Model file for the job. Use its own axes, mm. A direction names the side the tool comes from. Round coordinates to 2 decimals unless told otherwise and drop trailing zeros. Order: outer loops, then holes, each group sorted by start corner. A loop starts at its lowest first (then second) coordinate and runs counter-clockwise, first axis right, second up. Notation, with made-up numbers: (57.25, 86.5) - (70.25, 86.5) arc R20 ccw to (70.25, 120.5) - close; hole circle Ø1 at (75, -13). An arc over 180 degrees is marked (long way). Write item = value, one per line. Start each with the question number.
from build123d import *

# Parameters (mm, degrees)
F0_R     = 12.5
F1_DEPTH = 8.5
F2_R     = 10
F3_DEPTH = 5
F4_R     = 8
F5_DEPTH = 13.501
F6_SIZE  = 0.2


with BuildPart() as f1:
    # F0 (on Top) → F1 (new body)
    with BuildSketch(Plane.XY):
        Circle(F0_R)
    extrude(amount=F1_DEPTH)

    # F2 (on face) → F3 (join)
    with BuildSketch(Plane.XY.offset(8.5)):
        Circle(F2_R)
    extrude(amount=F3_DEPTH)

    # F4 (on face) → F5 (cut, through all)
    with BuildSketch(Plane.XY.offset(13.5)):
        Circle(F4_R)
    extrude(amount=-F5_DEPTH, mode=Mode.SUBTRACT)

    # F6
    f6_edges = [f1.edges().sort_by_distance(p)[0] for p in [
        (-10, 0, 13.5),
        (-8, 0, 13.5),
        (-12.5, 0, 8.5),
        (-10, 0, 8.5),
        (-12.5, 0, 0),
        (-8, 0, 0),
    ]]
    chamfer(f6_edges, length=F6_SIZE)


solid = f1.part
Item 1: Which spindle directions (+Z, -Z, +X, -X, +Y, -Y) get a long thin tool onto all of the face, cutting with end or side? Do faces 1 (the face through (-7.35, 7.35, 8.5)), 2 (the face through (-6, -6, 13.5)). Say none if no direction does.
Item 2: Mould opens along X. For faces 3 (the face through (8, -3, 0)), 4 (the face through (-1.73, -7.81, 6.84)), 5 (the face through (-2.17, -9.76, 10.97)) say: +X half, -X half, draft (parallel to the pull), parting line (faces both ways), or undercut.
Item 3: Drop flat-ended pins along their axis: pin 1 (6 mm diameter, centred on x = 10, z = 9.5, fed in from -Y); pin 2 (2 mm diameter, centred on x = 10, z = 9, fed in from +Y); pin 3 (5 mm diameter, centred on x = -9, z = 7, fed in from -Y). Give the stop position or say it passes through.
Item 4: Saw through at D-D, the plane z = 5.25. Give the cut face in (x, y).
Item 5: Probe L1, parallel to Y at x = 0, z = 4.75; L2, parallel to Y at x = 0, z = 8.75; L3, parallel to X at y = 4.25, z = 2.5. List the from-to ranges inside material, lowest first.
Item 6: Saw through at A-A, the plane y = 0. Give the cut face in (x, z), then the cut area to 3 significant figures.
Item 7: Saw through at C-C, the plane z = 11.5. Give the cut face in (x, y).
Check sheet entries:
q1.face_1 = +Z
q1.face_2 = +Z, +X, -X, +Y, -Y
q2.face_3 = draft
q2.face_4 = undercut
q2.face_5 = parting line
q3.pin_1 = -10.18
q3.pin_2 = 8.37
q3.pin_3 = -10.68
q4.outline = circle Ø25 at (0, 0); hole circle Ø16 at (0, 0)
q5.L1 = -12.5 to -8, 8 to 12.5
q5.L2 = -10 to -8, 8 to 10
q5.L3 = -11.76 to -6.78, 6.78 to 11.76
q6.outline = (-12.5, 0.2) - (-12.3, 0) - (-8.2, 0) - (-8, 0.2) - (-8, 13.3) - (-8.2, 13.5) - (-9.8, 13.5) - (-10, 13.3) - (-10, 8.7) - (-10.2, 8.5) - (-12.3, 8.5) - (-12.5, 8.3) - close; (8, 0.2) - (8.2, 0) - (12.3, 0) - (12.5, 0.2) - (12.5, 8.3) - (12.3, 8.5) - (10.2, 8.5) - (10, 8.7) - (10, 13.3) - (9.8, 13.5) - (8.2, 13.5) - (8, 13.3) - close
q6.area = 96.3 mm2
q7.outline = circle Ø20 at (0, 0); hole circle Ø16 at (0, 0)
